Geometry check sheet. Reference: the model listing, model coordinates, mm. A direction names the side the tool comes from. Round coordinates to 2 decimals unless told otherwise and drop trailing zeros. Loops run counter-clockwise (first coordinate to the right, second up) from the corner with the lowest first, then second, coordinate; pieces in that order, holes last.
```python
from build123d import *

# Parameters (mm, degrees)
F2_R           = 12.7
F3_DEPTH       = 12.701
F6_D           = 6.6
F6_CSINK_D     = 13.44
F6_CSINK_ANGLE = 90


# Not quite as in the source:
# - a length typed as a fraction of an inch, garbled in the dataset ("3 / 203.2 mm" for 3/8 in), is restored


with BuildPart() as f1:
    # F0 (on Front) → F1 (revolve)
    with BuildSketch(Plane.XZ):
        with BuildLine():
            Line((0, -46.4494958016), (0, 25.8821103648))
            ThreePointArc((0, 25.8821103648), (-8.9802561211, 22.1623664858), (-12.7, 13.1821103648))
            Line((-12.7, 13.1821103648), (-12.7, -25.4462463191))
            Line((-12.7, -25.4462463191), (-11.1125, -25.4462463191))
            Line((-11.1125, -25.4462463191), (-11.1125, -46.4494958016))
            Line((-11.1125, -46.4494958016), (0, -46.4494958016))
        make_face()
    revolve(axis=Axis((0, 0, -7.9082977027), (0, 0, -1)))

    # F2 (on Front) → F3 (cut, through all)
    with BuildSketch(Plane.XZ):
        with Locations((0, 13.1821103648)):
            Circle(F2_R)
    extrude(amount=-F3_DEPTH, mode=Mode.SUBTRACT)

    # F6 (through all)
    with Locations(Plane.XZ.offset(12.7)):
        with Locations((0, 13.1821103648)):
            CounterSinkHole(F6_D / 2, F6_CSINK_D / 2, counter_sink_angle=F6_CSINK_ANGLE)


solid = f1.part
```
1) Sectioned sample at D-D, the plane y = 9.5. Record the cut outline in (x, z), then the cut area to 3 significant figures.
Report:
outline: (-8.43, -25.45) - (-5.77, -25.45) - (-5.77, -46.45) - (5.77, -46.45) - (5.77, -25.45) - (8.43, -25.45) - (8.43, 3.68) arc R12.7 cw to (-8.43, 3.68) - close
area: 696 mm2
2) Mould release check, pull along Z, two halves, no side actions. Record for faces 4 (the face through (0.751, -9.446, 9.798)), 5 (the face through (-10.6, 3.34, -36.09)), 6 (the face through (-0.279, 4.85, 0.485)): +Z half, -Z half, draft (parallel to the pull), parting line (faces both ways), or undercut.
Report:
face 4: undercut
face 5: draft
face 6: +Z half
3) Sectioned sample at A-A, the plane x = 0. Record the cut outline in (y, z).
Report:
outline: (-12.7, -25.45) - (-11.11, -25.45) - (-11.11, -46.45) - (11.11, -46.45) - (11.11, -25.45) - (12.7, -25.45) - (12.7, 0.48) - (0, 0.48) - (0, 9.88) - (-9.28, 9.88) - (-12.7, 6.46) - close; (-11.46, 18.66) - (-9.28, 16.48) - (0, 16.48) - (0, 25.88) arc R12.7 ccw to start
4) Sectioned sample at C-C, the plane z = -28. Record the cut outline in (x, y) (1 decimal).
Report:
outline: circle Ø22.2 at (0, 0)
5) Gauge pin test, flat ends, axial feed: pin 1 (1 mm diameter, centred on x = -2, z = -19, fed in from -Y); pin 2 (6 mm diameter, centred on x = -7.5, y = -4.5, fed in from +Z); pin 3 (3 mm diameter, centred on x = -1.5, z = -34, fed in from -Y). Record the tip position at first contact, or that the pin passes through.
Report:
pin 1: stops at y = -12.61
pin 2: stops at z = 24.51
pin 3: stops at y = -11.11
6) Scan lines: line 1 along Z through (x, y) = (0, -2.5); line 2 along Z through (x, y) = (0, -5.25); line 3 along X through (y, z) = (-0.25, 11). Record each from-to range of solid material in increasing order.
Report:
line 1: z = -46.45 to 9.88, 16.48 to 25.63
line 2: z = -46.45 to 9.88, 16.48 to 24.75
line 3: x = -12.7 to -2.48, 2.48 to 12.7
7) Access from +Z, -Z, +X, -X, +Y, -Y to the whole of each face (thin tool, end or side, straight path). Record for faces 1 (the face through (0, 0, -46.449)), 2 (the face through (-0.88, -11.23, -25.446)), 3 (the face through (3, 0, 11)).
Report:
face 1: -Z, +X, -X, +Y, -Y
face 2: -Z
face 3: +Z, +Y
8) Sectioned sample at B-B, the plane y = -8.5. Record the cut outline in (x, z).
Report:
outline: (-9.44, -25.45) - (-7.16, -25.45) - (-7.16, -46.45) - (7.16, -46.45) - (7.16, -25.45) - (9.44, -25.45) - (9.44, 13.18) arc R9.44 ccw to (-9.44, 13.18) - close; hole circle Ø6.6 at (0, 13.18)
